Here's how the part is built. I have some questions about the finished solid (model axes, mm). Coordinates: 2 decimals unless noted, no trailing zeros. Order: outer loops, then holes, each group sorted by start corner. A loop starts at its lowest first (then second) coordinate and runs counter-clockwise, first axis right, second up. Notation, with made-up numbers: (75, -31.5) - (84, -31.5) arc R24 ccw to (84, 4.5) - close; hole circle Ø5 at (73.25, 68.25). An arc over 180 degrees is marked (long way). Answer as CSV lines item,"result". Start each with the question number.
Q1. Suppose I cut it at B-B (y = 7). Please give me the cut outline in (x, z).
Q2. For pin 1 Ø1 at (y, z) = (17.5, 1.5) entering from -X; pin 2 Ø3 at (x, y) = (4.5, 7) entering from -Z, each with a flat end and sliding along its axis, tell me the tip position at first contact or that it passes through.
Q3. Suppose I cut it at C-C (y = 37). Please give me the cut outline in (x, z).
Q4. Suppose I cut it at D-D (x = 4.5). Please give me the cut outline in (y, z).
Q5. Suppose I cut it at A-A (x = 72). Please give me the cut outline in (y, z), then the cut area to 3 significant figures.
Q6. I need wall thicknesses on line 1 (Y direction, x = 107.5, z = 1.25); line 2 (Y direction, x = 32, z = 1.9); line 3 (X direction, y = 46, z = 0.25). Which ranges of each line are inside material? Lowest first, please.
from build123d import *

# Parameters (mm, degrees)
SKETCH1_W           = 112
SKETCH1_H           = 70
BOSS_EXTRUDE1_DEPTH = 2
SKETCH2_W           = 98
SKETCH2_H           = 64.091260174
CUT_EXTRUDE1_DEPTH  = 133.090877808
SKETCH3_W           = 4
SKETCH3_H           = 46
CUT_EXTRUDE2_DEPTH  = 133.090877808
SKETCH4_R           = 1.75
SKETCH4_W           = 1
SKETCH4_H           = 4
CUT_EXTRUDE3_DEPTH  = 133.090877808


with BuildPart() as part:
    # Sketch1 → Boss-Extrude1 (new body)
    with BuildSketch(Plane.XY):
        with Locations((56, 35)):
            Rectangle(SKETCH1_W, SKETCH1_H)
    extrude(amount=BOSS_EXTRUDE1_DEPTH)

    # Sketch2 → Cut-Extrude1 (cut, through all)
    with BuildSketch(Plane.XY.offset(2)):
        with Locations((56, 34.954369913)):
            Rectangle(SKETCH2_W, SKETCH2_H)
    extrude(amount=-CUT_EXTRUDE1_DEPTH, mode=Mode.SUBTRACT)

    # Sketch3 → Cut-Extrude2 (cut, through all)
    with BuildSketch(Plane.XY.offset(2)):
        with Locations((5, 35)):
            Rectangle(SKETCH3_W, SKETCH3_H)
        with Locations((107, 35)):
            Rectangle(SKETCH3_W, SKETCH3_H)
    extrude(amount=-CUT_EXTRUDE2_DEPTH, mode=Mode.SUBTRACT)

    # Sketch4 → Cut-Extrude3 (cut, through all)
    with BuildSketch(Plane.XY.offset(2)):
        with Locations((4.5, 63)):
            Circle(SKETCH4_R)
        with Locations((4.5, 7)):
            Circle(SKETCH4_R)
        with Locations((107.5, 7)):
            Circle(SKETCH4_R)
        with Locations((107.5, 62.689831266)):
            Circle(SKETCH4_R)
        with Locations((2.5, 53)):
            Rectangle(SKETCH4_W, SKETCH4_H)
        with Locations((2.5, 17)):
            Rectangle(SKETCH4_W, SKETCH4_H)
        with Locations((109.5, 52.689831266)):
            Rectangle(SKETCH4_W, SKETCH4_H)
        with Locations((109.5, 17)):
            Rectangle(SKETCH4_W, SKETCH4_H)
    extrude(amount=-CUT_EXTRUDE3_DEPTH, mode=Mode.SUBTRACT)


solid = part.part
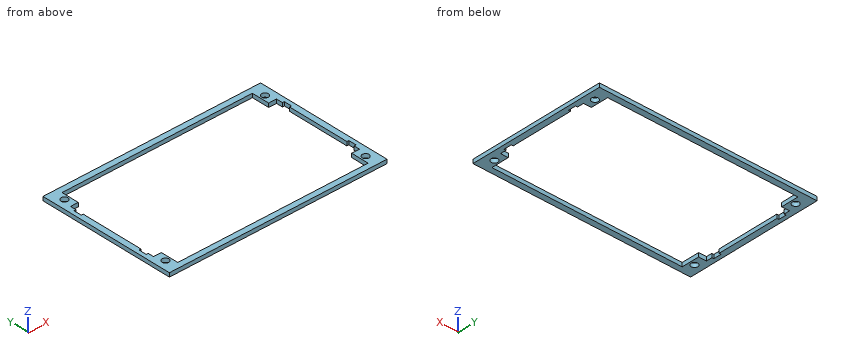
Here are the results:
1,outline,"(0, 0) - (2.75, 0) - (2.75, 2) - (0, 2) - close; (6.25, 0) - (7, 0) - (7, 2) - (6.25, 2) - close; (105, 0) - (105.75, 0) - (105.75, 2) - (105, 2) - close; (109.25, 0) - (112, 0) - (112, 2) - (109.25, 2) - close"
2,pin 1,"stops at x = 0"
2,pin 2,"passes through"
3,outline,"(0, 0) - (3, 0) - (3, 2) - (0, 2) - close; (109, 0) - (112, 0) - (112, 2) - (109, 2) - close"
4,outline,"(0, 0) - (5.25, 0) - (5.25, 2) - (0, 2) - close; (8.75, 0) - (12, 0) - (12, 2) - (8.75, 2) - close; (58, 0) - (61.25, 0) - (61.25, 2) - (58, 2) - close; (64.75, 0) - (70, 0) - (70, 2) - (64.75, 2) - close"
5,outline,"(0, 0) - (2.91, 0) - (2.91, 2) - (0, 2) - close; (67, 0) - (70, 0) - (70, 2) - (67, 2) - close"
5,area,"11.8 mm²"
6,line 1,"y = 0 to 5.25, 8.75 to 12, 58 to 60.94, 64.44 to 70"
6,line 2,"y = 0 to 2.91, 67 to 70"
6,line 3,"x = 0 to 3, 109 to 112"
